Model file for the job. Use its own axes, mm. A direction names the side the tool comes from. Round coordinates to 2 decimals unless told otherwise and drop trailing zeros. Loops run counter-clockwise (first coordinate to the right, second up) from the corner with the lowest first, then second, coordinate; pieces in that order, holes last. Notation, with made-up numbers: (68, 15) - (113, 15) arc R20 cw to (113, 19) - close; hole circle Ø11 at (63.5, 31.25). An arc over 180 degrees is marked (long way). Answer as a JSON object with one key per item and string values.
from build123d import *

# Parameters (mm, degrees)
SKETCH2_W           = 102
SKETCH2_H           = 89
BOSS_EXTRUDE1_DEPTH = 38
SKETCH3_R           = 24.13
BOSS_EXTRUDE2_DEPTH = 177.8
BOSS_EXTRUDE3_START = 50.8
SKETCH4_R           = 65
SKETCH4_R_2         = 63
BOSS_EXTRUDE3_DEPTH = 12
BOSS_EXTRUDE4_DEPTH = 2
SKETCH7_R           = 26.13
SKETCH7_R_2         = 24.13
BOSS_EXTRUDE6_DEPTH = 5
SKETCH6_R           = 3
BOSS_EXTRUDE5_DEPTH = 30
CHAMFER1_SIZE       = 4
CHAMFER1_SIZE2      = 2.309401077
FILLET1_R           = 4


with BuildPart() as part:
    # Sketch2 → Boss-Extrude1 (new body)
    with BuildSketch(Plane(origin=(0, 0, 0), x_dir=(1, 0, 0), z_dir=(0, 1, 0))):
        with Locations((6.5, 0)):
            Rectangle(SKETCH2_W, SKETCH2_H)
    extrude(amount=BOSS_EXTRUDE1_DEPTH)

    # Sketch3 → Boss-Extrude2 (add)
    with BuildSketch(Plane(origin=(0, 38, 0), x_dir=(1, 0, 0), z_dir=(0, 1, 0))):
        with Locations(Location((6.5, 0, 0), (0, 0, 270))):
            Circle(SKETCH3_R)
    extrude(amount=BOSS_EXTRUDE2_DEPTH)

    # Sketch5 → Boss-Extrude4 (add)
    with BuildSketch(Plane.XZ.offset(-88.8)):
        with BuildLine():
            Line((1.5, 23.606289416), (1.5, 62.801273872))
            ThreePointArc((1.5, 62.801273872), (6.5, 63), (11.5, 62.801273872))
            Line((11.5, 62.801273872), (11.5, 23.606289416))
            ThreePointArc((11.5, 23.606289416), (6.5, 24.13), (1.5, 23.606289416))
        make_face()
        with BuildLine():
            Line((69.301273872, -5), (30.106289416, -5))
            ThreePointArc((30.106289416, -5), (30.63, 0), (30.106289416, 5))
            Line((30.106289416, 5), (69.301273872, 5))
            ThreePointArc((69.301273872, 5), (69.5, 0), (69.301273872, -5))
        make_face()
        with BuildLine():
            Line((1.5, -62.801273872), (1.5, -23.606289416))
            ThreePointArc((1.5, -23.606289416), (6.5, -24.13), (11.5, -23.606289416))
            Line((11.5, -23.606289416), (11.5, -62.801273872))
            ThreePointArc((11.5, -62.801273872), (6.5, -63), (1.5, -62.801273872))
        make_face()
        with BuildLine():
            Line((-56.301273872, 5), (-17.106289416, 5))
            ThreePointArc((-17.106289416, 5), (-17.63, 0), (-17.106289416, -5))
            Line((-17.106289416, -5), (-56.301273872, -5))
            ThreePointArc((-56.301273872, -5), (-56.5, 0), (-56.301273872, 5))
        make_face()
    extrude(amount=-BOSS_EXTRUDE4_DEPTH)


with BuildPart() as body_2:
    # Sketch4 → Boss-Extrude3 (new body)
    with BuildSketch(Plane(origin=(0, 38, 0), x_dir=(1, 0, 0), z_dir=(0, 1, 0)).offset(BOSS_EXTRUDE3_START)):
        with Locations(Location((6.5, 0, 0), (0, 0, 270))):
            Circle(SKETCH4_R)
        with Locations(Location((6.5, 0, 0), (0, 0, 270))):
            Circle(SKETCH4_R_2, mode=Mode.SUBTRACT)
    extrude(amount=BOSS_EXTRUDE3_DEPTH)


    add(part.part)  # Boss-Extrude6 merges part
    # Sketch7 → Boss-Extrude6 (add)
    with BuildSketch(Plane.XZ.offset(-88.8)):
        with Locations(Location((6.5, 0, 0), (0, 0, 270))):
            Circle(SKETCH7_R)
        with Locations(Location((6.5, 0, 0), (0, 0, 90))):
            Circle(SKETCH7_R_2, mode=Mode.SUBTRACT)
    extrude(amount=-BOSS_EXTRUDE6_DEPTH)

    # Sketch6 → Boss-Extrude5 (add)
    with BuildSketch(Plane(origin=(0, 215.8, 0), x_dir=(1, 0, 0), z_dir=(0, 1, 0))):
        with Locations(Location((6.5, 0, 0), (0, 0, 270))):
            Circle(SKETCH6_R)
    extrude(amount=BOSS_EXTRUDE5_DEPTH)

    # Chamfer1
    chamfer1_edges = [body_2.edges().sort_by_distance(p)[0] for p in [
        (6.5, 245.8, -3),
    ]]
    chamfer1_side = [body_2.faces().sort_by_distance(p)[0] for p in [
        (6.5, 230.8, -3),
    ]]
    chamfer(chamfer1_edges, length=CHAMFER1_SIZE, length2=CHAMFER1_SIZE2, reference=chamfer1_side[0])

    # Fillet1
    fillet1_edges = [body_2.edges().sort_by_distance(p)[0] for p in [
        (-44.5, 0, 0),
        (-44.5, 19, -44.5),
        (6.5, 0, 44.5),
        (-44.5, 19, 44.5),
        (57.5, 0, 0),
        (57.5, 19, 44.5),
        (6.5, 0, -44.5),
        (57.5, 19, -44.5),
        (-44.5, 38, 0),
        (6.5, 38, 44.5),
        (57.5, 38, 0),
        (6.5, 38, -44.5),
    ]]
    fillet(fillet1_edges, radius=FILLET1_R)


solid = body_2.part
1) Slice it at B-B on y = 26. List the corners of the cut face in (x, z).
Values follow:
{"outline": "(-44.5, -40.5) arc R4 ccw to (-40.5, -44.5) - (53.5, -44.5) arc R4 ccw to (57.5, -40.5) - (57.5, 40.5) arc R4 ccw to (53.5, 44.5) - (-40.5, 44.5) arc R4 ccw to (-44.5, 40.5) - close"}
2) Drop flat-ended pins along their axis: P1, Ø0.6, axis at y = 90, z = 39.5, coming from the -X side; P2, Ø1, axis at x = 48, y = 89.5, coming from the +Z side; P3, Ø1, axis at x = -42, y = 89.5, coming from the -Z side. Give the stop position or say it passes through.
Values follow:
{"P1": "x = -45.35", "P2": "z = 50.44", "P3": "z = -43.83"}
3) Slice it at C-C on x = -50. List the corners of the cut face in (y, z), then the cut area to 3 significant figures.
Values follow:
{"outline": "(88.8, -32.14) - (100.8, -32.14) - (100.8, -27.87) - (88.8, -27.87) - close; (88.8, -5) - (90.8, -5) - (90.8, 5) - (88.8, 5) - close; (88.8, 27.87) - (100.8, 27.87) - (100.8, 32.14) - (88.8, 32.14) - close", "area": "122 mm²"}
4) Slice it at A-A on z = -7.5. List the corners of the cut face in (x, y), then the cut area to 3 significant figures.
Values follow:
{"outline": "(-58.07, 88.8) - (-56.05, 88.8) - (-56.05, 100.8) - (-58.07, 100.8) - close; (-44.5, 4) arc R4 ccw to (-40.5, 0) - (53.5, 0) arc R4 ccw to (57.5, 4) - (57.5, 34) arc R4 ccw to (53.5, 38) - (29.43, 38) - (29.43, 88.8) - (31.53, 88.8) - (31.53, 93.8) - (29.43, 93.8) - (29.43, 215.8) - (-16.43, 215.8) - (-16.43, 93.8) - (-18.53, 93.8) - (-18.53, 88.8) - (-16.43, 88.8) - (-16.43, 38) - (-40.5, 38) arc R4 ccw to (-44.5, 34) - close; (69.05, 88.8) - (71.07, 88.8) - (71.07, 100.8) - (69.05, 100.8) - close", "area": "12,100 mm²"}
5) Two-plate mould, pull along Z, no slides. Class faces 1 (the cylindrical face through (25.4, 94.7, 60.1)), 2 (the flat face through (6, 19, -44.5)), 3 (the cylindrical face through (3.57, 228.62, -0.65)), 4 (the flat face through (6, 38, -28)): pulls with the +Z half, pulls with the -Z half, needs draft (parallel to the pull), parting line crosses it, or undercut.
Values follow:
{"face 1": "undercut", "face 2": "pulls with the -Z half", "face 3": "parting line crosses it", "face 4": "needs draft"}
6) Tool access for faces 5 (the flat face through (6, 0, -1)), 6 (the flat face through (-38, 90.8, 0)), 7 (the cylindrical face through (13.748, 63.044, 23.016)): list every direction of +Z, -Z, +X, -X, +Y, -Y with a clear straight run to the whole face (end or side of a thin tool).
Values follow:
{"face 5": "+Z, -Z, +X, -X, -Y", "face 6": "+Y", "face 7": "none"}
7) Slice it at D-D on x = 38.5. List the corners of the cut face in (y, z).
Values follow:
{"outline": "(0, -40.5) arc R4 ccw to (4, -44.5) - (34, -44.5) arc R4 ccw to (38, -40.5) - (38, 40.5) arc R4 ccw to (34, 44.5) - (4, 44.5) arc R4 ccw to (0, 40.5) - close; (88.8, -56.58) - (100.8, -56.58) - (100.8, -54.27) - (88.8, -54.27) - close; (88.8, -5) - (90.8, -5) - (90.8, 5) - (88.8, 5) - close; (88.8, 54.27) - (100.8, 54.27) - (100.8, 56.58) - (88.8, 56.58) - close"}
8) Probe probe 1 along X at (y, z) = (93.5, 0); probe 2 along Z at (x, y) = (6, 93); probe 3 along X at (y, z) = (97.75, 0). List the from-to ranges inside material, lowest first.
Values follow:
{"probe 1": "-58.5 to -56.5, -19.63 to 32.63, 69.5 to 71.5", "probe 2": "-65 to -63, -26.13 to 26.13, 63 to 65", "probe 3": "-58.5 to -56.5, -17.63 to 30.63, 69.5 to 71.5"}
